Design review of the part shown in the three views and the two pictorial views. Dimensions are in mm from the part's minimum x, y and z. A direction names the side the tool comes from. Give positions to 0.01 mm unless a question says otherwise; leave off trailing zeros. Order: outer loops, then holes, each group sorted by start corner. A loop starts at its lowest first (then second) coordinate and runs counter-clockwise, first axis right, second up.
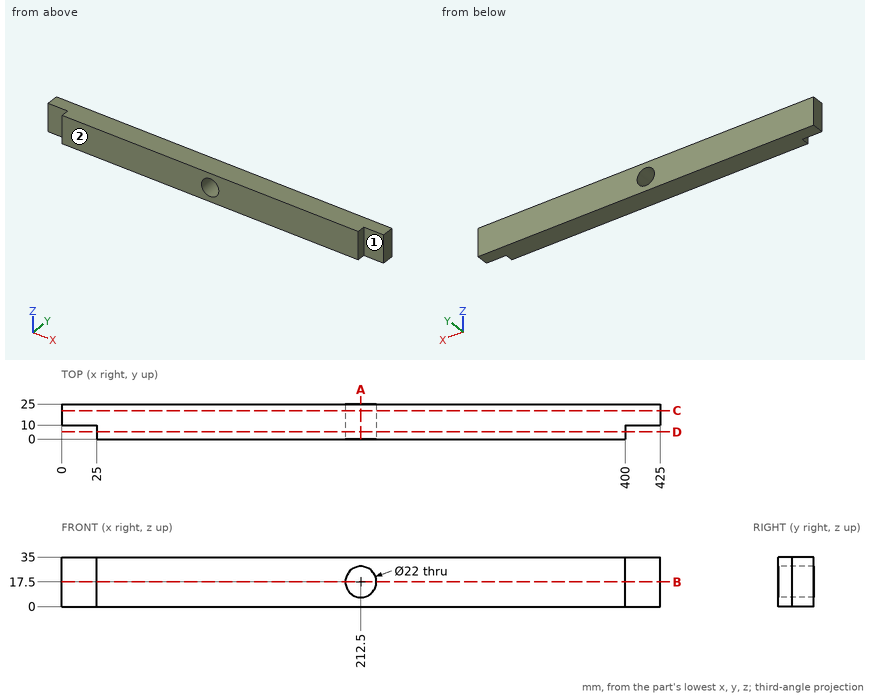
1) We need section C-C on y = 20.25. Give the boundary of the cut face in (x, z), then the cut area to 3 significant figures.
Answer sheet:
outline: (0, 0) - (425, 0) - (425, 35) - (0, 35) - close; hole circle Ø22 at (212.5, 17.5)
area: 14,500 mm2
2) To check wall thickness, follow line 1 (Z direction, x = 220.5, y = 22.25); line 2 (Z direction, x = 212.5, y = 6.5); line 3 (X direction, y = 1.75, z = 14.5). State the ranges of each line that lie inside material, in increasing order.
Answer sheet:
line 1: z = 0 to 9.95, 25.05 to 35
line 2: z = 0 to 6.5, 28.5 to 35
line 3: x = 25 to 201.92, 223.08 to 400
3) Tool access review of the marked faces 1 and 2: name each direction out of +Z, -Z, +X, -X, +Y, -Y from which nothing blocks a thin tool from reaching the whole face with its end or side.
Answer sheet:
face 1: +Z, -Z, +X, -Y
face 2: +Z, -Z, +X, -X, -Y
4) We need section B-B on z = 17.5. Give the boundary of the cut face in (x, y), then the cut area to 4 significant figures.
Answer sheet:
outline: (0, 10) - (25, 10) - (25, 0) - (201.5, 0) - (201.5, 25) - (0, 25) - close; (223.5, 0) - (400, 0) - (400, 10) - (425, 10) - (425, 25) - (223.5, 25) - close
area: 9,575 mm2
5) We need section A-A on x = 212.5. Give the boundary of the cut face in (y, z), then the cut area to 3 significant figures.
Answer sheet:
outline: (0, 0) - (25, 0) - (25, 6.5) - (0, 6.5) - close; (0, 28.5) - (25, 28.5) - (25, 35) - (0, 35) - close
area: 325 mm2
6) We need section D-D on y = 5.25. Give the boundary of the cut face in (x, z), then the cut area to 3 significant figures.
Answer sheet:
outline: (25, 0) - (400, 0) - (400, 35) - (25, 35) - close; hole circle Ø22 at (212.5, 17.5)
area: 12,700 mm2
7) Clearance check with flat-ended pins moving along their axes: pin 1 (5 mm diameter, centred on y = 3.5, z = 17, fed in from -X); pin 2 (7.5 mm diameter, centred on x = 17, z = 21, fed in from -Y); pin 3 (1.5 mm diameter, centred on x = 207.5, z = 24.5, fed in from +Y); pin 4 (3 mm diameter, centred on y = 5, z = 15.5, fed in from +X). State where each tip first meets the part, or that it passes through.
Answer sheet:
pin 1: stops at x = 25
pin 2: stops at y = 10
pin 3: passes through
pin 4: stops at x = 400
